Here's how the part is built. I have some questions about the finished solid (model axes, mm). A direction names the side the tool comes from. Coordinates: 2 decimals unless noted, no trailing zeros. Write each loop counter-clockwise with the first axis right and the second up, starting at its lowest first coordinate (ties: lowest second). Pieces come first, ordered by that corner, then holes. Notation, with made-up numbers: (31.5, -4) -> (57.5, -4) arc R21 cw to (57.5, 11) -> close; hole circle Ø10 at (54.25, 89). An arc over 180 degrees is marked (long way). Put each result on its own line as item: value.
```python
from build123d import *


with BuildPart() as part:
    # Esquisse1 → Révolution1 (revolve)
    with BuildSketch(Plane.XY, mode=Mode.PRIVATE) as r_volution1_sk:
        with BuildLine():
            Line((17, -6.5), (19.5, -6.5))
            Line((19.5, -6.5), (19.5, -4.5))
            Line((19.5, -4.5), (18, -4.5))
            Line((18, -4.5), (18, -1.936491673))
            ThreePointArc((18, -1.936491673), (16.777140216, -1.015753003), (16.563508327, 0.5))
            Line((16.563508327, 0.5), (15.383922662, 0.5))
            Line((15.383922662, 0.5), (17, -6.5))
        make_face()
    revolve(r_volution1_sk.sketch.rotate(Axis((0, -11.232892416, 0), (0, 1, 0)), 90), axis=Axis((0, -11.232892416, 0), (0, 1, 0)))  # turned: the seam where the file's is


solid = part.part
```
Item 1: Please list where these lines run through material, in increasing order: line 1 along Z through (x, y) = (-11, -4.75); line 2 along Z through (x, y) = (11, -5); line 3 along X through (y, z) = (-3, -14). Write a range as from..to.
Output:
line 1: z = -16.1..-12.43, 12.43..16.1
line 2: z = -16.1..-12.5, 12.5..16.1
line 3: x = -11.31..-8.14, 8.14..11.31
Item 2: For P1, Ø2, axis at y = -2, z = -14.5, coming from the +X side; P2, Ø1, axis at x = -3, y = -2.5, coming from the -Z side; P3, Ø1, axis at x = 13, y = -3.5, coming from the +Z side, each with a flat end and sliding along its axis, tell me the tip position at first contact or that it passes through.
Output:
P1: stops at x = 11.91
P2: stops at z = -17.83
P3: stops at z = 12.95
Item 3: Which directions (+Z, -Z, +X, -X, +Y, -Y) give clear straight access to the entire face, cutting with the end or side of a thin tool? Please do faces 4 (the cylindrical face through (-19.334, -5.486, 2.539)), 5 (the flat face through (17.24, -4.5, -5.69)).
Output:
face 4: +Y, -Y
face 5: +Y
Item 4: If we mould it in two halves opening along Z, with no side actions, what happens to faces 1 (the cylindrical face through (-12.165, -3.2, 13.267)), 2 (the flat face through (-17.4, -6.5, 1.4)), 3 (the conical face through (13.738, 0.062, -7.145))? For each: released by +Z, released by -Z, zero draft, split by the parting line, or undercut.
Output:
face 1: split by the parting line
face 2: zero draft
face 3: undercut
Item 5: Imagine slicing it at B-B on z = 0. Write out the boundary of the cut face in (x, y).
Output:
outline: (-19.5, -6.5) -> (-17, -6.5) -> (-15.38, 0.5) -> (-16.56, 0.5) arc R2 cw to (-18, -1.94) -> (-18, -4.5) -> (-19.5, -4.5) -> close; (15.38, 0.5) -> (17, -6.5) -> (19.5, -6.5) -> (19.5, -4.5) -> (18, -4.5) -> (18, -1.94) arc R2 cw to (16.56, 0.5) -> close
Item 6: Imagine slicing it at A-A on x = 0. Write out the boundary of the cut face in (y, z), then the cut area to 3 significant figures.
Output:
outline: (-6.5, -19.5) -> (-4.5, -19.5) -> (-4.5, -18) -> (-1.94, -18) arc R2 cw to (0.5, -16.56) -> (0.5, -15.38) -> (-6.5, -17) -> close; (-6.5, 17) -> (0.5, 15.38) -> (0.5, 16.56) arc R2 cw to (-1.94, 18) -> (-4.5, 18) -> (-4.5, 19.5) -> (-6.5, 19.5) -> close
area: 25.5 mm²
Item 7: Imagine slicing it at C-C on y = -3.5. Write out the boundary of the cut face in (x, z), then the cut area to 3 significant figures.
Output:
outline: circle Ø36 at (0, 0); hole circle Ø32.61 at (0, 0)
area: 182 mm²
